Can you work these out from the model? Positions are in its coordinate system, mm. A direction names the side the tool comes from. Give positions to 0.01 mm unless a question says otherwise; leave off trailing zeros. Loops run counter-clockwise (first coordinate to the right, second up) from the corner with the lowest first, then second, coordinate; pieces in that order, holes last. Notation, with made-up numbers: (88.5, -18) - (111.5, -18) arc R20 cw to (111.5, 8) - close; hole circle Ø8 at (33.5, -32). An arc over 180 degrees is marked (long way). Answer as a JSON object with one key per item and string values. Group by question number.
Item 1: Suppose I cut it at C-C on z = 3.25. Write out the boundary of the cut face in (x, y).
Item 2: Please list where these lines run through material, in increasing order: L1, parallel to Y at x = 45, z = 1; L2, parallel to Y at x = 25, z = 4.25; L3, parallel to X at y = 24.5, z = 3.5.
Item 3: Thinking about a two-plate mould opening in Y: for faces 1 (the flat face through (38, 33, 6.35)), 2 (the flat face through (49, 0, 3)), 3 (the flat face through (40.75, 33, 3)), 4 (the flat face through (51, 65, 3)), which applies, pulls with the +Y half, pulls with the -Y half, needs draft (parallel to the pull), parting line crosses it, or undercut?
Item 4: Which directions (+Z, -Z, +X, -X, +Y, -Y) give clear straight access to the entire face, cutting with the end or side of a thin tool? Please do faces 5 (the flat face through (64, 11.25, 3)), 6 (the flat face through (0, 33, 3)).
Item 5: Suppose I cut it at D-D on y = 15. Write out the boundary of the cut face in (x, z), and give its area (3 significant figures).
Item 6: Suppose I cut it at B-B on x = 74. Write out the boundary of the cut face in (y, z).
Item 7: Suppose I cut it at A-A on y = 32.5. Write out the boundary of the cut face in (x, z).
Item 8: Will this pin go through, and if not, where does the flat tip stop? pin 1 (20 mm diameter, centred on x = 25, y = 32.5, fed in from +Z).
Autodesk Inventor part; units mm, degrees
ref_plane "YZ Plane" through (0, 0, 0) normal (1, 0, 0) x (0, 1, 0)
ref_plane "XZ Plane" through (0, 0, 0) normal (0, 1, 0) x (-1, 0, 0)
ref_plane "XY Plane" through (0, 0, 0) normal (0, 0, 1) x (1, 0, 0)
sketch "Sketch1" plane through (0, 0, 0) normal (0, 0, 1) x (1, 0, 0)
  line L0 (0, 0) -> (100, 0)
  line L1 (100, 0) -> (100, 65)
  line L2 (100, 65) -> (0, 65)
  line L3 (0, 65) -> (0, 0)
  line L4 (88.25, 53.75) -> (40.75, 53.75)
  line L5 (40.75, 53.75) -> (40.75, 11.25)
  line L6 (40.75, 11.25) -> (88.25, 11.25)
  line L7 (88.25, 11.25) -> (88.25, 53.75)
  circle A0 centre (25, 32.5) radius 11.25
  point P0 (88.25, 32.5)
  point P1 (100, 32.5)
  point P2 (64.5, 53.75)
  dimension "d0" = 65
  dimension "d1" = 100
  dimension "d2" = 47.5
  dimension "d3" = 42.5
  dimension "d4" = 35.5
  dimension "d5" = 75
  dimension "d6" = 22.5
extrude "Extrusion1" add sketch "Sketch1" along normal blind 6.35
equation "\"d7\" = THICKB"
equation "\"THICKA\" = 3.175"
equation "\"THICKB\" = 6.35"
equation "\"THICKC\" = 12.7"
properties part number "WoodD_Extruder_Side_Hole"
Worked out:
{
 "1": {"outline": "(0, 0) - (100, 0) - (100, 65) - (0, 65) - close; hole circle Ø22.5 at (25, 32.5); hole (40.75, 11.25) - (88.25, 11.25) - (88.25, 53.75) - (40.75, 53.75) - close"},
 "2": {"L1": "y = 0 to 11.25, 53.75 to 65", "L2": "y = 0 to 21.25, 43.75 to 65", "L3": "x = 0 to 17.09, 32.91 to 40.75, 88.25 to 100"},
 "3": {"face 1": "needs draft", "face 2": "pulls with the -Y half", "face 3": "undercut", "face 4": "pulls with the +Y half"},
 "4": {"face 5": "+Z, -Z", "face 6": "+Z, -Z, -X, +Y, -Y"},
 "5": {"outline": "(0, 0) - (40.75, 0) - (40.75, 6.35) - (0, 6.35) - close; (88.25, 0) - (100, 0) - (100, 6.35) - (88.25, 6.35) - close", "area": "333 mm2"},
 "6": {"outline": "(0, 0) - (11.25, 0) - (11.25, 6.35) - (0, 6.35) - close; (53.75, 0) - (65, 0) - (65, 6.35) - (53.75, 6.35) - close"},
 "7": {"outline": "(0, 0) - (13.75, 0) - (13.75, 6.35) - (0, 6.35) - close; (36.25, 0) - (40.75, 0) - (40.75, 6.35) - (36.25, 6.35) - close; (88.25, 0) - (100, 0) - (100, 6.35) - (88.25, 6.35) - close"},
 "8": {"pin 1": "passes through"}
}
